Read the model definition and answer for the solid it produces. Units are mm, in the model's axes. A direction names the side the tool comes from. Round coordinates to 2 decimals unless told otherwise and drop trailing zeros. Order: outer loops, then holes, each group sorted by start corner. A loop starts at its lowest first (then second) coordinate and runs counter-clockwise, first axis right, second up. Notation, with made-up numbers: (80.5, -14.5) -> (129.5, -14.5) arc R22 ccw to (129.5, -0.5) -> close; hole circle Ø6 at (-35.75, -16.5). An arc over 180 degrees is marked (long way). Answer as a JSON object with one key per item and string values. Group by question number.
Item 1: Consider probe 1 along Z at (x, y) = (53.5, -26.5); probe 2 along X at (y, z) = (63, 38.5); probe 3 along Z at (x, y) = (4.5, -25). Determine where each line is inside the solid, lowest interval first. Write a range as from..to.
Item 2: Section B-B, the plane x = 5 is taken. Write down the section's boundary in (y, z), plus the area to 3 significant figures.
Item 3: Section C-C, the plane x = 35.5 is taken. Write down the section's boundary in (y, z).
Item 4: The mould has two halves that part along Z. Classify faces 1 (the flat face through (-27, 2, 22)), 2 (the flat face through (0, 2, -2)), 3 (the flat face through (-42, -2, 45)): pulls with the +Z half, pulls with the -Z half, needs draft (parallel to the pull), parting line crosses it, or undercut.
Item 5: Given P1, Ø2, axis at y = 25, z = 44, coming from the +X side; P2, Ø13, axis at y = 59.5, z = 24.5, coming from the -X side; P3, Ø6, axis at x = -32.5, y = 43.5, coming from the -Z side; P4, Ø3, axis at x = -24, z = 33.5, coming from the +Y side, each flat-ended and moving along its own axis, determine where each tip first touches the part or whether it passes through.
Item 6: Section A-A, the plane y = 10 is taken. Write down the section's boundary in (x, z), plus the area to 3 significant figures.
Item 7: For faces 4 (the flat face through (-51, -2, 42.9)), 5 (the flat face through (56, 2, 35.641)), 6 (the flat face through (57, 2, 33.641)), 7 (the flat face through (35.14, -2.1, 17.56)), determine the directions among +Z, -Z, +X, -X, +Y, -Y from which every point of the face is accessible in a straight line to the end or side of a thin tool.
from build123d import *

# Parameters (mm, degrees)
SCHIZZO2_W                     = 50
SCHIZZO2_H                     = 300
BASE_FLANGIA2_DEPTH            = 2
BORDO_FLANGIA1_STRIP_W         = 9.4732
BORDO_FLANGIA1_STRIP_H         = 2
BORDO_FLANGIA1_STRIP_CUT_DEPTH = 300
BORDO_FLANGIA1_DEPTH           = 300
BORDO_FLANGIA2_STRIP_W         = 9.4732
BORDO_FLANGIA2_STRIP_H         = 2
BORDO_FLANGIA2_STRIP_CUT_DEPTH = 300
BORDO_FLANGIA2_DEPTH           = 300
BORDO_FLANGIA3_STRIP_CUT_DEPTH = 300
BORDO_FLANGIA3_DEPTH           = 300
BORDO_FLANGIA4_STRIP_CUT_DEPTH = 300
BORDO_FLANGIA4_DEPTH           = 300
BORDO_FLANGIA5_STRIP_W         = 9.4732
BORDO_FLANGIA5_STRIP_H         = 2
BORDO_FLANGIA5_STRIP_CUT_DEPTH = 300
BORDO_FLANGIA5_DEPTH           = 300
ORLO1_START                    = -150
ORLO1_DEPTH                    = 300
ORLO1_2_DEPTH                  = 300


# Read off the part's stored shape, not the designer's step: Orlo1
# Sheet-metal steps are written as plain solids
with BuildPart() as part:
    # Schizzo2 → Base-Flangia2 (new body)
    with BuildSketch(Plane.XY):
        Rectangle(SCHIZZO2_W, SCHIZZO2_H)
    extrude(amount=-BASE_FLANGIA2_DEPTH)

    # Bordo-Flangia1 strip (across the edge) → Bordo-Flangia1 strip cut (cut)
    with BuildSketch(Plane(origin=(-25, 150, 0), x_dir=(1, 0, 0), z_dir=(0, -1, 0))):
        with Locations((-4, -1)):
            Rectangle(BORDO_FLANGIA1_STRIP_W, BORDO_FLANGIA1_STRIP_H)
    extrude(amount=BORDO_FLANGIA1_STRIP_CUT_DEPTH, mode=Mode.SUBTRACT)

    # Bordo-Flangia1 section (across the edge) → Bordo-Flangia1 (add)
    with BuildSketch(Plane(origin=(-25, 150, 0), x_dir=(1, 0, 0), z_dir=(0, -1, 0))):
        with BuildLine():
            Line((-2, 0.7366), (-2, 45))
            Line((-2, 45), (0, 45))
            Line((0, 45), (0, 0.7366))
            ThreePointArc((0, 0.7366), (0.215745145, 0.215745145), (0.7366, 0))
            Line((0.7366, 0), (0.7366, -2))
            ThreePointArc((0.7366, -2), (-1.198468417, -1.198468417), (-2, 0.7366))
        make_face()
    extrude(amount=BORDO_FLANGIA1_DEPTH)

    # Bordo-Flangia2 strip (across the edge) → Bordo-Flangia2 strip cut (cut)
    with BuildSketch(Plane(origin=(-27, -150, 45), x_dir=(0, 0, -1), z_dir=(0, 1, 0))):
        with Locations((-4, -1)):
            Rectangle(BORDO_FLANGIA2_STRIP_W, BORDO_FLANGIA2_STRIP_H)
    extrude(amount=BORDO_FLANGIA2_STRIP_CUT_DEPTH, mode=Mode.SUBTRACT)

    # Bordo-Flangia2 section (across the edge) → Bordo-Flangia2 (add)
    with BuildSketch(Plane(origin=(-27, -150, 45), x_dir=(0, 0, -1), z_dir=(0, 1, 0))):
        with BuildLine():
            Line((-2, 0.7366), (-2, 30))
            Line((-2, 30), (0, 30))
            Line((0, 30), (0, 0.7366))
            ThreePointArc((0, 0.7366), (0.215745145, 0.215745145), (0.7366, 0))
            Line((0.7366, 0), (0.7366, -2))
            ThreePointArc((0.7366, -2), (-1.198468417, -1.198468417), (-2, 0.7366))
        make_face()
    extrude(amount=BORDO_FLANGIA2_DEPTH)

    # Bordo-Flangia3 strip (across the edge) → Bordo-Flangia3 strip cut (cut)
    with BuildSketch(Plane(origin=(25, -150, 0), x_dir=(-0.8660254037844364, 0, 0.5000000000000041), z_dir=(0, 1, 0))):
        Polygon((-8.835731855, 2.791911088), (-0.6317, -1.944688912), (0.3683, -0.212638104), (-7.835731855, 4.523961896), align=None)
    extrude(amount=BORDO_FLANGIA3_STRIP_CUT_DEPTH, mode=Mode.SUBTRACT)

    # Bordo-Flangia3 section (across the edge) → Bordo-Flangia3 (add)
    with BuildSketch(Plane(origin=(25, -150, 0), x_dir=(-0.8660254037844364, 0, 0.5000000000000041), z_dir=(0, 1, 0))):
        with BuildLine():
            Line((-2, 0.425276208), (-2, 40))
            Line((-2, 40), (0, 40))
            Line((0, 40), (0, 0.425276208))
            ThreePointArc((0, 0.425276208), (0.098685688, 0.056976208), (0.3683, -0.212638104))
            Line((0.3683, -0.212638104), (-0.6317, -1.944688912))
            ThreePointArc((-0.6317, -1.944688912), (-1.63336512, -0.943023792), (-2, 0.425276208))
        make_face()
    extrude(amount=BORDO_FLANGIA3_DEPTH)

    # Bordo-Flangia4 strip (across the edge) → Bordo-Flangia4 strip cut (cut)
    with BuildSketch(Plane(origin=(46.732050808, 150, 33.641016151), x_dir=(0, 0, -1), z_dir=(0, -1, 0))):
        Polygon((-8.835731855, 2.791911088), (-0.6317, -1.944688912), (0.3683, -0.212638104), (-7.835731855, 4.523961896), align=None)
    extrude(amount=BORDO_FLANGIA4_STRIP_CUT_DEPTH, mode=Mode.SUBTRACT)

    # Bordo-Flangia4 section (across the edge) → Bordo-Flangia4 (add)
    with BuildSketch(Plane(origin=(46.732050808, 150, 33.641016151), x_dir=(0, 0, -1), z_dir=(0, -1, 0))):
        with BuildLine():
            Line((-2, 0.425276208), (-2, 20))
            Line((-2, 20), (0, 20))
            Line((0, 20), (0, 0.425276208))
            ThreePointArc((0, 0.425276208), (0.098685688, 0.056976208), (0.3683, -0.212638104))
            Line((0.3683, -0.212638104), (-0.6317, -1.944688912))
            ThreePointArc((-0.6317, -1.944688912), (-1.63336512, -0.943023792), (-2, 0.425276208))
        make_face()
    extrude(amount=BORDO_FLANGIA4_DEPTH)

    # Bordo-Flangia5 strip (across the edge) → Bordo-Flangia5 strip cut (cut)
    with BuildSketch(Plane(origin=(66.732050808, 150, 33.641016151), x_dir=(-1, 0, 0), z_dir=(0, -1, 0))):
        with Locations((-4, -1)):
            Rectangle(BORDO_FLANGIA5_STRIP_W, BORDO_FLANGIA5_STRIP_H)
    extrude(amount=BORDO_FLANGIA5_STRIP_CUT_DEPTH, mode=Mode.SUBTRACT)

    # Bordo-Flangia5 section (across the edge) → Bordo-Flangia5 (add)
    with BuildSketch(Plane(origin=(66.732050808, 150, 33.641016151), x_dir=(-1, 0, 0), z_dir=(0, -1, 0))):
        with BuildLine():
            Line((-2, 0.7366), (-2, 12))
            Line((-2, 12), (0, 12))
            Line((0, 12), (0, 0.7366))
            ThreePointArc((0, 0.7366), (0.215745145, 0.215745145), (0.7366, 0))
            Line((0.7366, 0), (0.7366, -2))
            ThreePointArc((0.7366, -2), (-1.198468417, -1.198468417), (-2, 0.7366))
        make_face()
    extrude(amount=BORDO_FLANGIA5_DEPTH)

    # Orlo1 outline → Orlo1 (cut)
    with BuildSketch(Plane(origin=(0, 0, 0), x_dir=(1, 0, 0), z_dir=(0, 1, 0)).offset(ORLO1_START)):
        with BuildLine():
            ThreePointArc((-54.95, -47), (-56.381782106, -46.417140075), (-56.999390153, -45))
            Line((-56.999390153, -45), (-57, -45))
            Line((-57, -45), (-57, -47))
            Line((-57, -47), (-54.95, -47))
        make_face()
    extrude(amount=ORLO1_DEPTH, mode=Mode.SUBTRACT)

    # Orlo1 2 outline → Orlo1 2 (add)
    with BuildSketch(Plane(origin=(0, 0, 0), x_dir=(1, 0, 0), z_dir=(0, 1, 0)).offset(ORLO1_START)):
        with BuildLine():
            Line((-47, -44.9), (-47, -42.9))
            Line((-47, -42.9), (-54.95, -42.9))
            ThreePointArc((-54.95, -42.9), (-56.417140075, -43.518217894), (-56.999390153, -45))
            Line((-56.999390153, -45), (-54.95, -45))
            ThreePointArc((-54.95, -45), (-55, -44.95), (-54.95, -44.9))
            Line((-54.95, -44.9), (-47, -44.9))
        make_face()
    extrude(amount=ORLO1_2_DEPTH)


solid = part.part
Values found:
{
 "1": {"probe 1": "33.64..35.64", "probe 2": "-27..-25", "probe 3": "-2..0"},
 "2": {"outline": "(-150, -2) -> (150, -2) -> (150, 0) -> (-150, 0) -> close", "area": "600 mm2"},
 "3": {"outline": "(-150, 14.19) -> (150, 14.19) -> (150, 18.19) -> (-150, 18.19) -> close"},
 "4": {"face 1": "needs draft", "face 2": "pulls with the -Z half", "face 3": "undercut"},
 "5": {"P1": "x = -25", "P2": "x = -27", "P3": "z = 45", "P4": "y = 150"},
 "6": {"outline": "(-54.95, 42.9) -> (-47, 42.9) -> (-47, 44.9) -> (-54.95, 44.9) arc R0.05 cw to (-54.95, 45) -> (-27.74, 45) arc R0.74 cw to (-27, 44.26) -> (-27, 0.74) arc R2.74 ccw to (-24.26, -2) -> (24.57, -2) arc R2.74 ccw to (26.94, -0.63) -> (46.52, 33.27) arc R0.74 cw to (47.16, 33.64) -> (66, 33.64) arc R0.74 cw to (66.73, 32.9) -> (66.73, 21.64) -> (68.73, 21.64) -> (68.73, 32.9) arc R2.74 ccw to (66, 35.64) -> (47.16, 35.64) arc R2.74 ccw to (44.79, 34.27) -> (25.21, 0.37) arc R0.74 cw to (24.57, 0) -> (-24.26, 0) arc R0.74 cw to (-25, 0.74) -> (-25, 44.26) arc R2.74 ccw to (-27.74, 47) -> (-54.95, 47) arc R2.05 ccw to start", "area": "424 mm2"},
 "7": {"face 4": "-Z, -X, +Y, -Y", "face 5": "+Z, +X, +Y, -Y", "face 6": "-Z, +Y, -Y", "face 7": "+Z, +Y, -Y"}
}
